Work out the finished part from the listing and answer in its coordinate system (mm). Face numbers are marked on the shaded views. A direction names the side the tool comes from. Coordinates: 2 decimals unless noted, no trailing zeros. Loops run counter-clockwise (first coordinate to the right, second up) from the corner with the lowest first, then second, coordinate; pieces in that order, holes last. Notation, with made-up numbers: (83, 52) - (130, 52) arc R28 ccw to (130, 73) - close; hole circle Ø5 at (-12, -26.5). An arc over 180 degrees is marked (long way). Write each question's results on one line, items separated by ' | '. Start each with the question number.
Item 1: Section B-B, the plane x = 0.5 is taken. Write down the section's boundary in (y, z).
Item 2: Section A-A, the plane y = 0 is taken. Write down the section's boundary in (x, z).
Item 3: A tool of negligible diameter and unlimited length cuts with its end or side. For the marked faces 5, 6, 7 and 8, from which of +Z, -Z, +X, -X, +Y, -Y can it reach the whole face along a straight path? Write none if from no direction.
Item 4: Section C-C, the plane z = -5.5 is taken. Write down the section's boundary in (x, y) (3 decimals), plus the area to 3 significant figures.
Item 5: For a pull along X with two mould halves and no side action, classify the marked faces 1, 2, 3 and 4 as +X half, -X half, draft (parallel to the pull), parting line (faces both ways), or undercut.
Item 6: Consider probe 1 along Y at (x, z) = (12.7, -4.5); probe 2 along X at (y, z) = (-8.5, -6); probe 3 along Y at (x, z) = (-2.5, -6). Determine where each line is inside the solid, lowest interval first. Write a range as [from, to].
Item 7: Section D-D, the plane y = -14.75 is taken. Write down the section's boundary in (x, z).
Item 8: Each of these flat-tipped pins is pushed along its axis until it touches: pin 1 Ø0.5 at (y, z) = (-17, -2.5) entering from +X; pin 2 Ø4 at (x, y) = (12.7, -9.398) entering from -Z; pin 3 Ø2 at (x, z) = (-0.5, -4) entering from -Y; pin 4 Ø1 at (y, z) = (-7, -6.5) entering from +X. Where does it stop, or does it pass through?
from build123d import *

# Parameters (mm, degrees)
SKETCH1_R           = 1.1938
BOSS_EXTRUDE1_DEPTH = 7.7724


with BuildPart() as part:
    # Sketch1 → Boss-Extrude1 (new body)
    with BuildSketch(Plane.XY):
        with BuildLine():
            Line((-5.065262452, 5.08), (-18.456556559, 5.08))
            ThreePointArc((-18.456556559, 5.08), (-19.426909517, 4.731155792), (-19.953034117, 3.844324324))
            ThreePointArc((-19.953034117, 3.844324324), (-18.44069754, -8.534815418), (-9.9822, -17.699098371))
            Line((-9.9822, -17.699098371), (-9.9822, -16.784328658))
            Line((-9.9822, -16.784328658), (2.593084415, -20.153865962))
            ThreePointArc((2.593084415, -20.153865962), (10.900004065, -17.149119843), (17.146958643, -10.903403565))
            Line((17.146958643, -10.903403565), (12.940315476, -3.61728387))
            ThreePointArc((12.940315476, -3.61728387), (12.796393961, -3.475289825), (12.60008731, -3.426922378))
            ThreePointArc((12.60008731, -3.426922378), (9.17217903, -2.398369889), (7.028137334, 0.467212181))
            Line((7.028137334, 0.467212181), (6.053096787, 3.371693793))
            ThreePointArc((6.053096787, 3.371693793), (1.669604011, 7.303273092), (-3.95481445, 5.560217822))
            ThreePointArc((-3.95481445, 5.560217822), (-4.460344292, 5.205196933), (-5.065262452, 5.08))
        make_face()
        with Locations((12.7, -9.398)):
            Circle(SKETCH1_R, mode=Mode.SUBTRACT)
        with BuildLine():
            Line((-3.876453526, 1.038692592), (-3.482013301, 2.510763551))
            ThreePointArc((-3.482013301, 2.510763551), (-2.298514325, 4.447599489), (-0.253578298, 5.432607064))
            Line((-0.253578298, 5.432607064), (-0.201054745, 5.628627633))
            ThreePointArc((-0.201054745, 5.628627633), (-0.082709585, 5.782858048), (0.110030452, 5.808232755))
            Line((0.110030452, 5.808232755), (2.808827211, 5.085092343))
            ThreePointArc((2.808827211, 5.085092343), (2.963057626, 4.966747183), (2.988432333, 4.774007146))
            Line((2.988432333, 4.774007146), (2.93590878, 4.577986577))
            ThreePointArc((2.93590878, 4.577986577), (4.214371541, 2.702476981), (4.270893751, 0.433378367))
            Line((4.270893751, 0.433378367), (3.876453526, -1.038692592))
            ThreePointArc((3.876453526, -1.038692592), (-1.038692592, -3.876453526), (-3.876453526, 1.038692592))
        make_face(mode=Mode.SUBTRACT)
    extrude(amount=-BOSS_EXTRUDE1_DEPTH)


solid = part.part
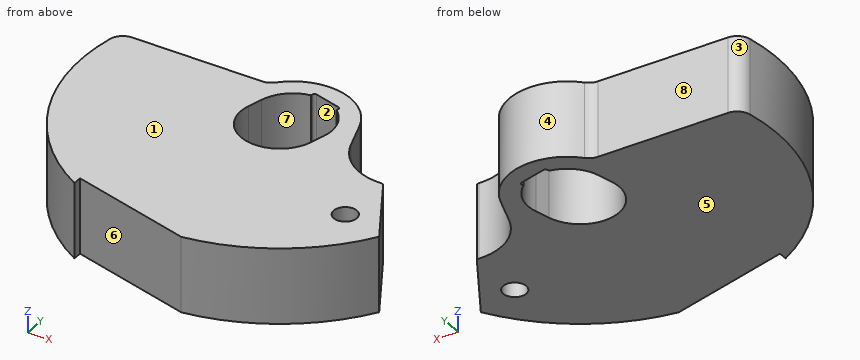
Answer key:
1) outline: (-19.59, -7.77) - (-3.98, -7.77) - (-3.98, 0) - (-19.59, 0) - close; (5.7, -7.77) - (7.44, -7.77) - (7.44, 0) - (5.7, 0) - close
2) outline: (-20.32, -7.77) - (-4.01, -7.77) - (-4.01, 0) - (-20.32, 0) - close; (4.15, -7.77) - (7.21, -7.77) - (7.21, 0) - (4.15, 0) - close
3) face 5: -Z, +X, -X, +Y, -Y | face 6: +Z, -Z, -Y | face 7: +Z, -Z | face 8: +Z, -Z, -X, +Y
4) outline: (-19.953, 3.844) arc R20.32 ccw to (-9.982, -17.699) - (-9.982, -16.784) - (2.593, -20.154) arc R20.32 ccw to (17.147, -10.903) - (12.94, -3.617) arc R0.381 ccw to (12.6, -3.427) arc R5.715 cw to (7.028, 0.467) - (6.053, 3.372) arc R5.969 ccw to (-3.955, 5.56) arc R1.524 cw to (-5.065, 5.08) - (-18.457, 5.08) arc R1.524 ccw to start; hole (-3.876, 1.039) arc R4.013 ccw to (3.876, -1.039) - (4.271, 0.433) arc R4.013 ccw to (2.936, 4.578) - (2.988, 4.774) arc R0.254 ccw to (2.809, 5.085) - (0.11, 5.808) arc R0.254 ccw to (-0.201, 5.629) - (-0.254, 5.433) arc R4.013 ccw to (-3.482, 2.511) - close; hole circle Ø2.388 at (12.7, -9.398) | area: 647 mm^2
5) face 1: draft | face 2: undercut | face 3: -X half | face 4: parting line
6) probe 1: y = [-15.86, -10.59], [-8.2, -3.44] | probe 2: x = [-18.46, 11.91], [13.49, 15.76] | probe 3: y = [-18.79, -3.14], [4.25, 6.69]
7) outline: (-13.98, -7.77) - (13.98, -7.77) - (13.98, 0) - (-13.98, 0) - close
8) pin 1: stops at x = 11.5 | pin 2: stops at z = -7.77 | pin 3: stops at y = -19.59 | pin 4: stops at x = 15.18
